```python
from build123d import *

# Parameters (mm, degrees)
BOSS_EXTRUDE1_DEPTH = 10
SKETCH2_R           = 6.75
BOSS_EXTRUDE2_DEPTH = 18.2
SKETCH3_R           = 4
BOSS_EXTRUDE3_DEPTH = 10
SKETCH4_R           = 4
CUT_EXTRUDE1_DEPTH  = 26.4


with BuildPart() as part:
    # Sketch1 → Boss-Extrude1 (new body)
    with BuildSketch(Plane(origin=(0, 0, 0), x_dir=(1, 0, 0), z_dir=(0, 1, 0))):
        Polygon((0, 9.237604307), (-8, 4.618802154), (-8, -4.618802154), (0, -9.237604307), (8, -4.618802154), (8, 4.618802154), align=None)
    extrude(amount=BOSS_EXTRUDE1_DEPTH)

    # Sketch2 → Boss-Extrude2 (add)
    with BuildSketch(Plane(origin=(0, 10, 0), x_dir=(1, 0, 0), z_dir=(0, 1, 0))):
        Circle(SKETCH2_R)
    extrude(amount=BOSS_EXTRUDE2_DEPTH)

    # Sketch3 → Boss-Extrude3 (add)
    with BuildSketch(Plane.XZ):
        Circle(SKETCH3_R)
    extrude(amount=BOSS_EXTRUDE3_DEPTH)

    # Sketch4 → Cut-Extrude1 (cut)
    with BuildSketch(Plane(origin=(0, 28.2, 0), x_dir=(1, 0, 0), z_dir=(0, 1, 0))):
        Circle(SKETCH4_R)
    extrude(amount=-CUT_EXTRUDE1_DEPTH, mode=Mode.SUBTRACT)


solid = part.part
```
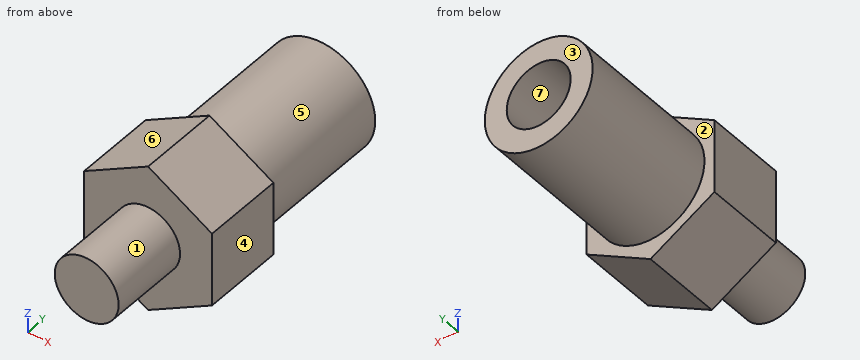
Check sheet for the modelled part. Datum: model origin and axes. Units: mm. Face numbers are marked on the shaded views. A direction names the side the tool comes from. Round coordinates to 2 decimals unless told otherwise and drop trailing zeros. Order: outer loops, then holes, each group sorted by start corner. A loop starts at its lowest first (then second) coordinate and runs counter-clockwise, first axis right, second up. Notation, with made-up numbers: (37, 0.25) -> (93, 0.25) arc R25 ccw to (93, 19.25) -> close; hole circle Ø10 at (21.5, -36). An arc over 180 degrees is marked (long way). Use CSV: the item, a comma, the result in double quotes.
(1) Depth check by flat-ended pin: pin 1 (5 mm diameter, centred on y = -5.5, z = 2, fed in from -X); pin 2 (1.5 mm diameter, centred on x = 5, z = -6.5, fed in from -Y); pin 3 (4 mm diameter, centred on x = 6, y = 15.5, fed in from -Z). Enter the tip coordinate at first touch or a pass-through.
Worked out:
pin 1,"x = -4"
pin 2,"y = 0"
pin 3,"z = -5.44"
(2) Cross-section at A-A (y = 9). Record the boundary of the cut face in (x, z), and give its area (3 significant figures).
Worked out:
outline,"(-8, -4.62) -> (0, -9.24) -> (8, -4.62) -> (8, 4.62) -> (0, 9.24) -> (-8, 4.62) -> close; hole circle Ø8 at (0, 0)"
area,"171 mm²"
(3) Cross-section at D-D (z = 8). Record the boundary of the cut face in (x, y), and give its area (3 significant figures).
Worked out:
outline,"(-2.14, 0) -> (2.14, 0) -> (2.14, 10) -> (-2.14, 10) -> close"
area,"42.9 mm²"
(4) Cross-section at B-B (z = 0). Record the boundary of the cut face in (x, y).
Worked out:
outline,"(-8, 0) -> (-4, 0) -> (-4, -10) -> (4, -10) -> (4, 0) -> (8, 0) -> (8, 10) -> (6.75, 10) -> (6.75, 28.2) -> (4, 28.2) -> (4, 1.8) -> (-4, 1.8) -> (-4, 28.2) -> (-6.75, 28.2) -> (-6.75, 10) -> (-8, 10) -> close"
(5) Material ranges on line 1 along X through (y, z) = (18.5, 0); line 2 along Z through (x, y) = (0, 8.25), recorded low to high. Write a range as from..to.
Worked out:
line 1,"-6.75..-4, 4..6.75"
line 2,"-9.24..-4, 4..9.24"
(6) Cross-section at C-C (x = 2.5). Record the boundary of the cut face in (y, z), and give its area (3 significant figures).
Worked out:
outline,"(-10, -3.12) -> (0, -3.12) -> (0, -7.79) -> (10, -7.79) -> (10, -6.27) -> (28.2, -6.27) -> (28.2, -3.12) -> (1.8, -3.12) -> (1.8, 3.12) -> (28.2, 3.12) -> (28.2, 6.27) -> (10, 6.27) -> (10, 7.79) -> (0, 7.79) -> (0, 3.12) -> (-10, 3.12) -> close"
area,"282 mm²"
(7) Tool access check on the marked faces 1, 2 and 3. Record the directions out of +Z, -Z, +X, -X, +Y, -Y that give a thin tool (end or side, any length) a straight path to the whole face; none if there is none.
Worked out:
face 1,"-Y"
face 2,"+Y"
face 3,"+Z, -Z, +X, -X, +Y"
(8) Draft check along Z on the marked faces 4, 5, 6 and 7. Enter one of: pulls with the +Z half, pulls with the -Z half, needs draft (parallel to the pull), parting line crosses it, or undercut.
Worked out:
face 4,"needs draft"
face 5,"parting line crosses it"
face 6,"pulls with the +Z half"
face 7,"undercut"
